Check sheet for the modelled part. Datum: model origin and axes. Units: mm. A direction names the side the tool comes from. Give positions to 0.01 mm unless a question says otherwise; leave off trailing zeros. Order: outer loops, then holes, each group sorted by start corner. A loop starts at its lowest first (then second) coordinate and runs counter-clockwise, first axis right, second up. Notation, with made-up numbers: (21.5, 35.5) -> (46.5, 35.5) arc R24 ccw to (46.5, 64.5) -> close; hole circle Ø3 at (-25, 70.25). An arc over 180 degrees is marked (long way). Answer in a Markdown table with one row per item. Add a question column.
(1) Cross-section at A-A (z = 8). Record the cut outline in (x, y), then the cut area to 3 significant figures.
(2) Cross-section at B-B (x = -47). Record the cut outline in (y, z), then the cut area to 3 significant figures.
(3) Set-up check for faces 5 (the face through (-50.332, 16.768, 36.099)), 6 (the face through (-61.471, 28, 22)): record each of +Z, -Z, +X, -X, +Y, -Y from which the full face is reachable in a straight line by a thin tool's end or side.
(4) Go/stop test with flat-tipped pins: pin 1 (14 mm diameter, centred on x = -44.5, z = 26.5, fed in from +Y); pin 2 (3.5 mm diameter, centred on y = 31.78, z = 22.5, fed in from +X). Record where each tip stops, or that it passes through.
(5) Cross-section at D-D (y = 19.5). Record the cut outline in (x, z).
(6) Cross-section at C-C (z = 22.5). Record the cut outline in (x, y), then the cut area to 3 significant figures.
(7) Thickness scan on L1, parallel to X at y = 17.25, z = 37; L2, parallel to Y at x = -54, z = 38; L3, parallel to X at y = 40, z = 36. Record the ranges inside material, lowest first. Write a range as [from, to].
(8) Release check for a two-part mould opening along Y. For faces 1 (the face through (-33.471, 17, 22)), 2 (the face through (-62, 45.782, 22)), 3 (the face through (-49, 15.782, 22)), 4 (the face through (-62.48, 33.27, 22.3)) record: released by +Y, released by -Y, zero draft, split by the parting line, or undercut.
```python
from build123d import *

# Parameters (mm, degrees)
P_IDAT_VYSUNUT_M1_DEPTH       = 45
D_RY_PRO_KOL_K_VELIKOST_MM1_D = 6
D_RY_PRO_KOL_K_VELIKOST_MM2_D = 3


with BuildPart() as part:
    # Skica1 → Přidat vysunutím1 (new body)
    with BuildSketch(Plane.XY):
        Polygon((-63.470895832, 45.782217357), (-63.470895832, 15.782217357), (-33.470895832, 15.782217357), (-33.470895832, 17.782217357), (-61.470895832, 17.782217357), (-61.470895832, 45.782217357), align=None)
    extrude(amount=P_IDAT_VYSUNUT_M1_DEPTH)

    # Díry pro kolík, velikost mm1 (through all)
    with Locations(Plane(origin=(0, 17.782217357, 0), x_dir=(1, 0, 0), z_dir=(0, 1, 0))):
        with Locations((-47.470895832, -37), (-47.470895832, -8)):
            Hole(D_RY_PRO_KOL_K_VELIKOST_MM1_D / 2)

    # Díry pro kolík, velikost mm2 (through all)
    with Locations(Plane(origin=(-61.470895832, 0, 0), x_dir=(0, 0, -1), z_dir=(1, 0, 0))):
        with Locations((-22.5, 31.782217357)):
            Hole(D_RY_PRO_KOL_K_VELIKOST_MM2_D / 2)


solid = part.part
```
Answer below:
| question | item | result |
|---|---|---|
| 1 | outline | (-63.47, 15.78) -> (-50.47, 15.78) -> (-50.47, 17.78) -> (-61.47, 17.78) -> (-61.47, 45.78) -> (-63.47, 45.78) -> close; (-44.47, 15.78) -> (-33.47, 15.78) -> (-33.47, 17.78) -> (-44.47, 17.78) -> close |
| 1 | area | 104 mm² |
| 2 | outline | (15.78, 0) -> (17.78, 0) -> (17.78, 5.04) -> (15.78, 5.04) -> close; (15.78, 10.96) -> (17.78, 10.96) -> (17.78, 34.04) -> (15.78, 34.04) -> close; (15.78, 39.96) -> (17.78, 39.96) -> (17.78, 45) -> (15.78, 45) -> close |
| 2 | area | 66.3 mm² |
| 3 | face 5 | +Y, -Y |
| 3 | face 6 | +Z, -Z, +X, +Y |
| 4 | pin 1 | stops at y = 17.78 |
| 4 | pin 2 | stops at x = -61.47 |
| 5 | outline | (-63.47, 0) -> (-61.47, 0) -> (-61.47, 45) -> (-63.47, 45) -> close |
| 6 | outline | (-63.47, 15.78) -> (-33.47, 15.78) -> (-33.47, 17.78) -> (-61.47, 17.78) -> (-61.47, 30.28) -> (-63.47, 30.28) -> close; (-63.47, 33.28) -> (-61.47, 33.28) -> (-61.47, 45.78) -> (-63.47, 45.78) -> close |
| 6 | area | 110 mm² |
| 7 | L1 | x = [-63.47, -50.47], [-44.47, -33.47] |
| 7 | L2 | y = [15.78, 17.78] |
| 7 | L3 | x = [-63.47, -61.47] |
| 8 | face 1 | zero draft |
| 8 | face 2 | released by +Y |
| 8 | face 3 | released by -Y |
| 8 | face 4 | undercut |
